```python
from build123d import *

# Parameters (mm, degrees)
SKETCH1_W           = 48
SKETCH1_H           = 48
BOSS_EXTRUDE1_DEPTH = 16
SKETCH2_R           = 4
CUT_EXTRUDE1_DEPTH  = 100
SKETCH3_R           = 3.75
BOSS_EXTRUDE2_DEPTH = 10
FILLET1_R           = 5
CHAMFER1_SIZE       = 3


with BuildPart() as part:
    # Sketch1 → Boss-Extrude1 (new body)
    with BuildSketch(Plane(origin=(0, 0, 0), x_dir=(1, 0, 0), z_dir=(0, 1, 0))):
        Rectangle(SKETCH1_W, SKETCH1_H)
    extrude(amount=BOSS_EXTRUDE1_DEPTH)

    # Sketch2 → Cut-Extrude1 (cut)
    with BuildSketch(Plane.XY.offset(24)):
        with Locations((-15, 8)):
            Circle(SKETCH2_R)
        with Locations((15, 8)):
            Circle(SKETCH2_R)
    extrude(amount=-CUT_EXTRUDE1_DEPTH, mode=Mode.SUBTRACT)

    # Sketch3 → Boss-Extrude2 (add)
    with BuildSketch(Plane(origin=(24, 0, 0), x_dir=(0, 0, -1), z_dir=(1, 0, 0))):
        with Locations(Location((0, 8, 0), (0, 0, 180))):
            Circle(SKETCH3_R)
    boss_extrude2 = extrude(amount=BOSS_EXTRUDE2_DEPTH)

    # Mirror1: Boss-Extrude2 across plane
    add(boss_extrude2.mirror(Plane(origin=(0, 0, 0), x_dir=(0, 0, 1), z_dir=(1, 0, 0))))

    # Fillet1
    fillet1_edges = [part.edges().sort_by_distance(p)[0] for p in [
        (24, 8, 24),
        (-24, 8, 24),
        (-24, 8, -24),
        (24, 8, -24),
    ]]
    fillet(fillet1_edges, radius=FILLET1_R - 0.0001)  # a hair under: the kernel refuses the full size

    # Chamfer1
    chamfer1_edges = [part.edges().sort_by_distance(p)[0] for p in [
        (0, 16, -24),
        (24, 16, 0),
        (-24, 16, 0),
        (0, 16, 24),
        (-22.535563195, 16, 22.535563195),
        (-22.535563195, 16, -22.535563195),
        (22.535563195, 16, 22.535563195),
        (22.535563195, 16, -22.535563195),
    ]]
    chamfer(chamfer1_edges, length=CHAMFER1_SIZE)


solid = part.part
```
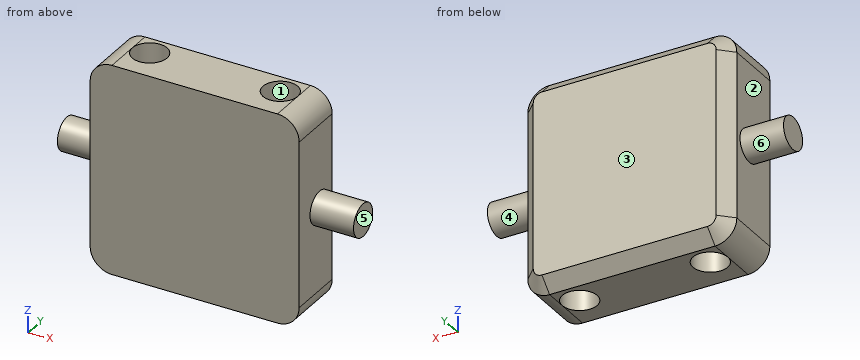
Here's how the part is built. I have some questions about the finished solid (model axes, mm). Face numbers are marked on the shaded views. A direction names the side the tool comes from. Round coordinates to 2 decimals unless told otherwise and drop trailing zeros. Order: outer loops, then holes, each group sorted by start corner. A loop starts at its lowest first (then second) coordinate and runs counter-clockwise, first axis right, second up. Notation, with made-up numbers: M 68,32.25 L 96,32.25 A24 ccw 96,48.25 Z; hole C -39.75,-27 d4. An arc over 180 degrees is marked long. Answer in a Markdown table with one row per item.
Item 1: For the marked faces 4, 5 and 6, which set-ups out of +Z, -Z, +X, -X, +Y, -Y let a thin tool reach every point of the face, with its end or its side?
A:
| item | result |
|---|---|
| face 4 | +X |
| face 5 | +Z, -Z, +X, +Y, -Y |
| face 6 | -X |
Item 2: Imagine slicing it at A-A, the plane y = 8. State how many separate pieces and enclosed holes the cut face has, and give its area (3 significant figures).
A:
| item | result |
|---|---|
| separate pieces | 3 |
| enclosed holes | 0 |
| area | 1,660 mm2 |
Item 3: Thinking about a two-plate mould opening in X: for the marked faces 1, 2 and 3, which applies, +X half, -X half, draft (parallel to the pull), parting line (faces both ways), or undercut?
A:
| item | result |
|---|---|
| face 1 | undercut |
| face 2 | -X half |
| face 3 | draft |
Item 4: I'm going to push flat-ended pins straight in: pin 1 (1 mm diameter, centred on x = 7, z = 0, fed in from -Y); pin 2 (1.5 mm diameter, centred on y = 6, z = 14, fed in from +X); pin 3 (6.5 mm diameter, centred on x = -15, y = 8, fed in from +Z). Where does each tip first touch, or does it pass through?
A:
| item | result |
|---|---|
| pin 1 | stops at y = 0 |
| pin 2 | stops at x = 24 |
| pin 3 | passes through |
Item 5: If I drill on L1, parallel to Y at x = 15, z = 2.5; L2, parallel to X at y = 7.75, z = 2; L3, parallel to X at y = 9, z = 14.5, over which ranges is the centre line in solid material (lowest first)? Write a range as from..to.
A:
| item | result |
|---|---|
| L1 | y = 0..4, 12..16 |
| L2 | x = -34..-18.99, -11.01..11.01, 18.99..34 |
| L3 | x = -24..-18.87, -11.13..11.13, 18.87..24 |
Item 6: Imagine slicing it at D-D, the plane z = 3. Write out the boundary of the cut face in (x, y).
A:
| item | result |
|---|---|
| outline | M -34,5.75 L -24,5.75 L -24,0 L 24,0 L 24,5.75 L 34,5.75 L 34,10.25 L 24,10.25 L 24,13 L 21,16 L -21,16 L -24,13 L -24,10.25 L -34,10.25 Z; hole C -15,8 d8; hole C 15,8 d8 |
Item 7: Imagine slicing it at C-C, the plane z = 17. Write out the boundary of the cut face in (x, y).
A:
| item | result |
|---|---|
| outline | M -24,0 L 24,0 L 24,13 L 21,16 L -21,16 L -24,13 Z; hole C -15,8 d8; hole C 15,8 d8 |
Item 8: Imagine slicing it at B-B, the plane x = -15. Write out the boundary of the cut face in (y, z), and give its area (3 significant figures).
A:
| item | result |
|---|---|
| outline | M 0,-24 L 4,-24 L 4,24 L 0,24 Z; M 12,-24 L 13,-24 L 16,-21 L 16,21 L 13,24 L 12,24 Z |
| area | 375 mm2 |
